Design review of the part shown in the three views and the two pictorial views. Dimensions are in mm from the part's minimum x, y and z. Give positions to 0.01 mm unless a question says otherwise; leave off trailing zeros. Loops run counter-clockwise (first coordinate to the right, second up) from the corner with the lowest first, then second, coordinate; pieces in that order, holes last. Notation, with made-up numbers: (-28.5, -4.5) - (17.5, -4.5) arc R18 ccw to (17.5, 16.5) - close; hole circle Ø11 at (58.25, -1.5). An arc over 180 degrees is marked (long way). Answer as a JSON object with one key per item and string values.
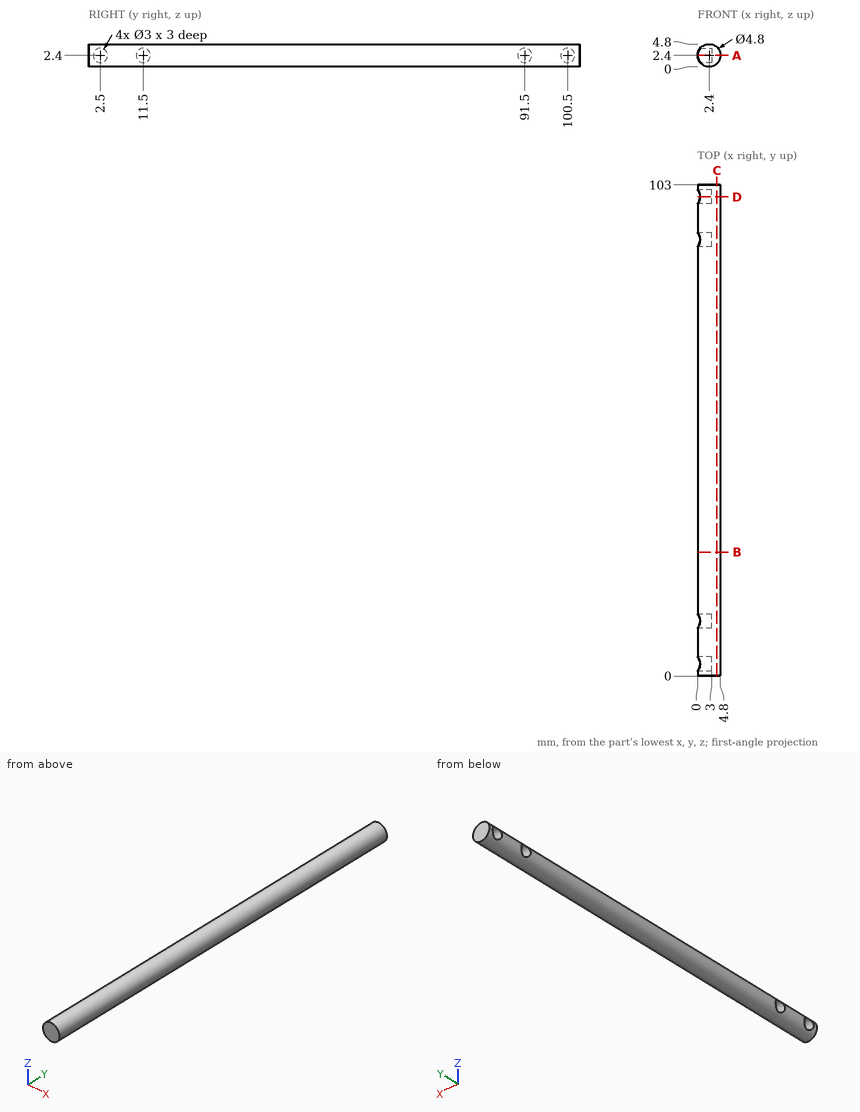
Q1. To check wall thickness, follow probe 1 along Y at (x, z) = (1.4, 2.4); probe 2 along Y at (x, z) = (2, 1.45); probe 3 along X at (y, z) = (68.5, 2.05). State the ranges of each line that lie inside material, in increasing order. Write a range as [from, to].
Results:
{"probe 1": "y = [0, 1], [4, 10], [13, 90], [93, 99], [102, 103]", "probe 2": "y = [0, 1.34], [3.66, 10.34], [12.66, 90.34], [92.66, 99.34], [101.66, 103]", "probe 3": "x = [0.03, 4.77]"}
Q2. Clearance check with flat-ended pins moving along their axes: pin 1 Ø1.5 at (y, z) = (101, 2) entering from -X; pin 2 Ø2 at (y, z) = (21.5, 1) entering from -X. State where each tip first meets the part, or that it passes through.
Results:
{"pin 1": "stops at x = 3", "pin 2": "stops at x = 0.03"}
Q3. Consider section D-D, the plane y = 100.5. State the section outline as (x, z) points, plus the area to 3 significant figures.
Results:
{"outline": "(0.53, 0.9) arc R2.4 ccw (long way) to (0.53, 3.9) - (3, 3.9) - (3, 0.9) - close", "area": "9.60 mm^2"}
Q4. Consider section B-B, the plane y = 26. State the section outline as (x, z) points, plus the area to 3 significant figures.
Results:
{"outline": "circle Ø4.8 at (2.4, 2.4)", "area": "18.1 mm^2"}
Q5. Consider section A-A, the plane z = 2.4. State the section outline as (x, y) points.
Results:
{"outline": "(0, 0) - (4.8, 0) - (4.8, 103) - (0, 103) - (0, 102) - (3, 102) - (3, 99) - (0, 99) - (0, 93) - (3, 93) - (3, 90) - (0, 90) - (0, 13) - (3, 13) - (3, 10) - (0, 10) - (0, 4) - (3, 4) - (3, 1) - (0, 1) - close"}
Q6. Consider section C-C, the plane x = 4.05. State the section outline as (y, z) points, plus the area to 3 significant figures.
Results:
{"outline": "(0, 0.66) - (103, 0.66) - (103, 4.14) - (0, 4.14) - close", "area": "359 mm^2"}
